Input: part model. Units: mm. Frame: model coordinates. Face numbers are marked on the shaded views. A direction names the side the tool comes from. Round coordinates to 2 decimals unless told otherwise and drop trailing zeros. Loops run counter-clockwise (first coordinate to the right, second up) from the corner with the lowest first, then second, coordinate; pieces in that order, holes last.
(1) Cut plane A-A, the plane z = -16. Output: boundary loops of the cut face in (x, y).
(2) First-contact query: pin 1 Ø8 at (x, y) = (58, 10) entering from +Z; pin 2 Ø9 at (x, z) = (26, -19.5) entering from +Y; pin 3 Ø10 at (x, z) = (46, -34.5) entering from +Y. Flat tips, straight axial feed; report the tip coordinate or a pass-through.
(3) Cut plane D-D, the plane z = -25.5. Output: boundary loops of the cut face in (x, y), and give its area (3 significant figures).
(4) Draft query along X for the marked faces 6, 7 and 8. Return one class per face: released by +X, released by -X, zero draft, split by the parting line, or undercut.
(5) Access query for the marked faces 1, 2, 3, 4 and 5. Directions: +Z, -Z, +X, -X, +Y, -Y. A direction counts if a zero-diameter tool reaches every point of the face in a straight line with its end or side. Return the directions, or none.
(6) Cut plane C-C, the plane y = 12. Output: boundary loops of the cut face in (x, z), and give its area (3 significant figures).
(7) Line query: line 1 (Y direction, x = 60, z = -6.25); line 2 (X direction, y = 48, z = -46); line 3 (X direction, y = 15.5, z = -12). Output: solid intervals per line, ascending.
(8) Cut plane B-B, the plane x = 60. Output: boundary loops of the cut face in (y, z), and give its area (3 significant figures).
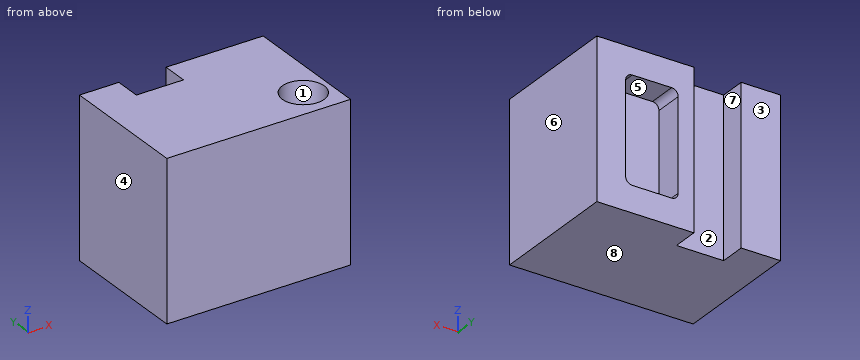
from build123d import *

# Parameters (mm, degrees)
ESBO_O7_W                                      = 70
ESBO_O7_H                                      = 50
RESSALTO_EXTRUS_O3_DEPTH                       = 60
BROCA_DE_ROSQUEAR_PARA_TARRAXA_DE_M1_2X0_D     = 16
BROCA_DE_ROSQUEAR_PARA_TARRAXA_DE_M1_2X0_DEPTH = 22
CORTE_EXTRUS_O2_DEPTH                          = 11
ESBO_O13_W                                     = 18
ESBO_O13_H                                     = 10


with BuildPart() as part:
    # Esboço7 → Ressalto-extrusão3 (new body)
    with BuildSketch(Plane.XY):
        with Locations((35, 25)):
            Rectangle(ESBO_O7_W, ESBO_O7_H)
    extrude(amount=-RESSALTO_EXTRUS_O3_DEPTH)

    # Broca de rosquear para tarraxa de M1.2x0.252
    with Locations(Plane.XY):
        with Locations((60, 12)):
            Hole(BROCA_DE_ROSQUEAR_PARA_TARRAXA_DE_M1_2X0_D / 2, depth=BROCA_DE_ROSQUEAR_PARA_TARRAXA_DE_M1_2X0_DEPTH)

    # Esboço11 → Corte-extrusão2 (cut)
    with BuildSketch(Plane(origin=(0, 50, 0), x_dir=(1, 0, 0), z_dir=(0, 1, 0))):
        with BuildLine():
            Line((41.5, 50), (56.5, 50))
            ThreePointArc((56.5, 50), (58.267766953, 49.267766953), (59, 47.5))
            Line((59, 47.5), (59, 12.5))
            ThreePointArc((59, 12.5), (58.267766953, 10.732233047), (56.5, 10))
            Line((56.5, 10), (41.5, 10))
            ThreePointArc((41.5, 10), (39.732233047, 10.732233047), (39, 12.5))
            Line((39, 12.5), (39, 47.5))
            ThreePointArc((39, 47.5), (39.732233047, 49.267766953), (41.5, 50))
        make_face()
    extrude(amount=-CORTE_EXTRUS_O2_DEPTH, mode=Mode.SUBTRACT)

    # Varredura de corte1: sweep along a path in Esboço16
    with BuildLine(Plane(origin=(0, 50, 0), x_dir=(1, 0, 0), z_dir=(0, 1, 0))) as varredura_de_corte1_path:
        Line((15, 0), (15, 60))
    # Esboço13 → Varredura de corte1 (sweep, cut)
    with BuildSketch(Plane.XY):
        with Locations((24, 45)):
            Rectangle(ESBO_O13_W, ESBO_O13_H)
    sweep(path=varredura_de_corte1_path.line, mode=Mode.SUBTRACT)


solid = part.part
Reported:
1. outline: (0, 0) - (70, 0) - (70, 50) - (59, 50) - (59, 39) - (39, 39) - (39, 50) - (33, 50) - (33, 40) - (15, 40) - (15, 50) - (0, 50) - close; hole circle Ø16 at (60, 12)
2. pin 1: stops at z = -22
2. pin 2: stops at y = 40
2. pin 3: stops at y = 39
3. outline: (0, 0) - (70, 0) - (70, 50) - (59, 50) - (59, 39) - (39, 39) - (39, 50) - (33, 50) - (33, 40) - (15, 40) - (15, 50) - (0, 50) - close
3. area: 3,100 mm2
4. face 6: released by +X
4. face 7: undercut
4. face 8: zero draft
5. face 1: +Z
5. face 2: +Z, -Z, +Y
5. face 3: +Z, -Z, +X, -X, +Y
5. face 4: +Z, -Z, -X, +Y, -Y
5. face 5: +Y
6. outline: (0, -60) - (70, -60) - (70, 0) - (68, 0) - (68, -22) - (52, -22) - (52, 0) - (0, 0) - close
6. area: 3,850 mm2
7. line 1: y = 0 to 4, 20 to 50
7. line 2: x = 0 to 15, 33 to 39, 59 to 70
7. line 3: x = 0 to 52.81, 67.19 to 70
8. outline: (0, -60) - (50, -60) - (50, 0) - (20, 0) - (20, -22) - (4, -22) - (4, 0) - (0, 0) - close
8. area: 2,650 mm2
